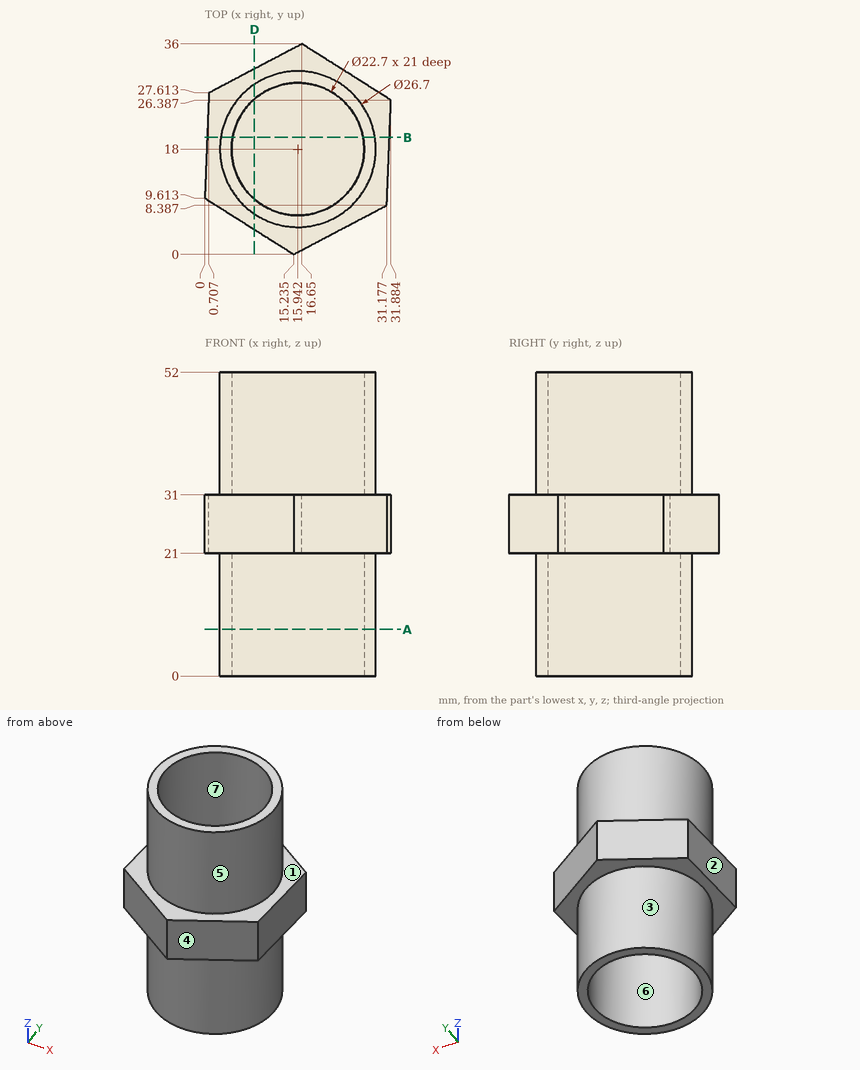
Print and shaded views of the part. All mm, measured from the part's lowest x, y and z. A direction names the side the tool comes from. Coordinates: 2 decimals unless noted, no trailing zeros. Write each loop counter-clockwise with the first axis right and the second up, starting at its lowest first coordinate (ties: lowest second). Pieces come first, ordered by that corner, then holes.
(1) Cut at D-D, the plane x = 8.5. List the corners of the cut face in (y, z), and give its area (3 significant figures).
(2) Cut at A-A, the plane z = 8. List the corners of the cut face in (x, y), and give its area (3 significant figures).
(3) Cut at B-B, the plane y = 20. List the corners of the cut face in (x, z) (1 decimal).
(4) Flat gauge pins, fed straight in: pin 1 (10 mm diameter, centred on x = 23, z = 10, fed in from -Y); pin 2 (1 mm diameter, centred on x = 15.5, y = 17, fed in from +Z); pin 3 (2 mm diameter, centred on x = 18.5, z = 12, fed in from +Y). Where does each tip first touch, or does it go through?
(5) Two-plate mould, pull along Y, no slides. Class the marked faces 4, 5, 6 and 7: +Y half, -Y half, draft (parallel to the pull), parting line (faces both ways), or undercut.
(6) Drill centre lines: probe 1 along Z at (x, y) = (1, 17); probe 2 along Y at (x, z) = (9, 50.5) (1 decimal); probe 3 along X at (y, z) = (25, 31.5) (1 decimal). Where is each one in solid material? Low to high.
(7) 3-axis set-ups, long thin cutter, end or side, ignore diameter. For the marked faces 1, 2 and 3: which of +Z, -Z, +X, -X, +Y, -Y reach the whole face in a straight line?
Geometry says:
1. outline: (4.25, 21) - (6.92, 21) - (6.92, 0) - (9.43, 0) - (9.43, 21) - (26.57, 21) - (26.57, 0) - (29.08, 0) - (29.08, 21) - (31.71, 21) - (31.71, 31) - (29.08, 31) - (29.08, 52) - (26.57, 52) - (26.57, 31) - (9.43, 31) - (9.43, 52) - (6.92, 52) - (6.92, 31) - (4.25, 31) - close
1. area: 486 mm2
2. outline: circle Ø26.7 at (15.94, 18); hole circle Ø22.7 at (15.94, 18)
2. area: 155 mm2
3. outline: (0.4, 21) - (2.7, 21) - (2.7, 0) - (4.8, 0) - (4.8, 21) - (27.1, 21) - (27.1, 0) - (29.1, 0) - (29.1, 21) - (31.6, 21) - (31.6, 31) - (29.1, 31) - (29.1, 52) - (27.1, 52) - (27.1, 31) - (4.8, 31) - (4.8, 52) - (2.7, 52) - (2.7, 31) - (0.4, 31) - close
4. pin 1: stops at y = 4.81
4. pin 2: stops at z = 31
4. pin 3: stops at y = 31.26
5. face 4: -Y half
5. face 5: parting line
5. face 6: undercut
5. face 7: undercut
6. probe 1: z = 21 to 31
6. probe 2: y = 6.6 to 9, 27 to 29.4
6. probe 3: x = 4.6 to 7, 24.9 to 27.3
7. face 1: +Z
7. face 2: +Z, -Z, -X, +Y
7. face 3: -Z
